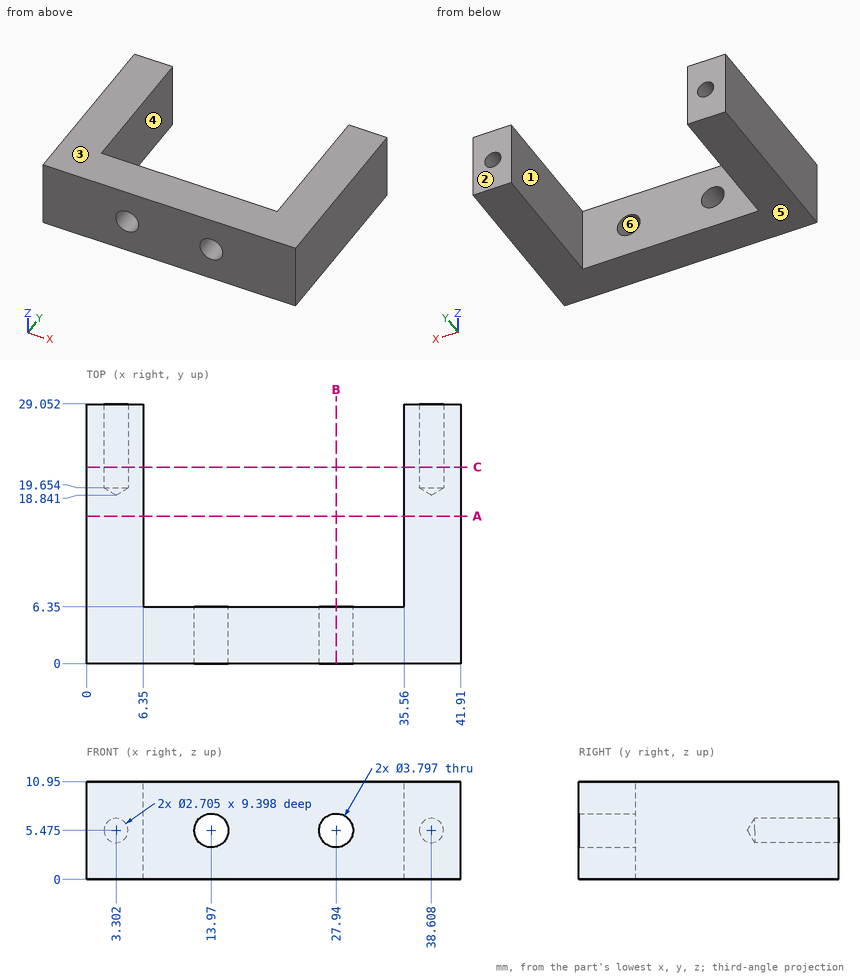
Drawing for the job (mm, zero at the part's lowest x, y, z). A direction names the side the tool comes from. Give positions to 0.01 mm unless a question says otherwise; leave off trailing zeros. Loops run counter-clockwise (first coordinate to the right, second up) from the corner with the lowest first, then second, coordinate; pieces in that order, holes last. Notation, with made-up numbers: M 85,25 L 108,25 A22 cw 108,36 Z; hole C 60.25,55 d8. An arc over 180 degrees is marked long. Use one line per item in the form item = value.
Item 1: Two-plate mould, pull along Z, no slides. Class the marked faces 3, 4, 5 and 6: pulls with the +Z half, pulls with the -Z half, needs draft (parallel to the pull), parting line crosses it, or undercut.
Determined:
face_3 = pulls with the +Z half
face_4 = needs draft
face_5 = pulls with the -Z half
face_6 = undercut
Item 2: Which spindle directions (+Z, -Z, +X, -X, +Y, -Y) get a long thin tool onto all of the face, cutting with end or side? Do the marked faces 1 and 2. Say none if no direction does.
Determined:
face_1 = +Z, -Z, +Y
face_2 = +Z, -Z, +X, -X, +Y
Item 3: Slice it at A-A (y = 16.5). List the corners of the cut face in (x, z), plus the area to 3 significant figures.
Determined:
outline = M 0,0 L 6.35,0 L 6.35,10.95 L 0,10.95 Z; M 35.56,0 L 41.91,0 L 41.91,10.95 L 35.56,10.95 Z
area = 139 mm2
Item 4: Drill centre lines: probe 1 along X at (y, z) = (22.5, 4); probe 2 along Z at (x, y) = (27.94, 3); probe 3 along X at (y, z) = (26.5, 6.25). Where is each one in solid material? Low to high. Write a range as from..to.
Determined:
probe_1 = 0..6.35, 35.56..41.91
probe_2 = 0..3.58, 7.37..10.95
probe_3 = 0..2.19, 4.41..6.35, 35.56..37.5, 39.72..41.91
Item 5: Flat gauge pins, fed straight in: pin 1 (4 mm diameter, centred on x = 32.5, y = 20.5, fed in from -Z); pin 2 (5 mm diameter, centred on x = 19.5, z = 5, fed in from +Y); pin 3 (2 mm diameter, centred on x = 38.608, z = 5.475, fed in from +Y). Where does each tip first touch, or does it go through?
Determined:
pin_1 = through
pin_2 = 6.35
pin_3 = 19.44
Item 6: Slice it at C-C (y = 22). Count the separate pieces of the cut face and the enclosed holes in it, plus the area to 3 significant figures.
Determined:
separate_pieces = 2
enclosed_holes = 2
area = 128 mm2
Item 7: Slice it at B-B (x = 27.94). List the corners of the cut face in (y, z).
Determined:
outline = M 0,0 L 6.35,0 L 6.35,3.58 L 0,3.58 Z; M 0,7.37 L 6.35,7.37 L 6.35,10.95 L 0,10.95 Z
